The model under review builds one solid part; all positions refer to its coordinate system, in mm. Face numbers are marked on the shaded views. A direction names the side the tool comes from. Give positions to 0.01 mm unless a question says otherwise; leave off trailing zeros. Order: outer loops, then holes, each group sorted by start corner. A loop starts at its lowest first (then second) coordinate and runs counter-clockwise, first axis right, second up.
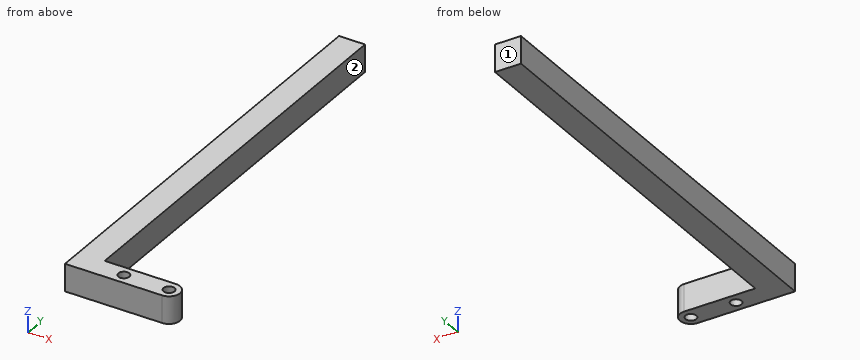
```python
from build123d import *

# Parameters (mm, degrees)
SKETCH_1_R      = 1
EXTRUDE_1_DEPTH = 5


with BuildPart() as part:
    # 草图1 → 凸台-拉伸1 (new body)
    with BuildSketch(Plane.XY):
        with BuildLine():
            Line((0, 2), (8.25, 2))
            ThreePointArc((8.25, 2), (10.25, 0), (8.25, -2))
            Line((8.25, -2), (-0.5, -2))
            Line((-0.5, -2), (-9.5, -2))
            Line((-9.5, -2), (-9.5, 78))
            Line((-9.5, 78), (-4.75, 78))
            Line((-4.75, 78), (-4.75, 2))
            Line((-4.75, 2), (0, 2))
        make_face()
        Circle(SKETCH_1_R, mode=Mode.SUBTRACT)
        with Locations((8.25, 0)):
            Circle(SKETCH_1_R, mode=Mode.SUBTRACT)
    extrude(amount=EXTRUDE_1_DEPTH)


solid = part.part
```
1. Take a section at C-C (z = 1.4). Write out the cut boundary in (x, y).
2. Take a section at D-D (x = 4.5). Write out the cut boundary in (y, z), and give its area (3 significant figures).
3. Insertion check: pin 1 (3 mm diameter, centred on y = 42, z = 2.5, fed in from +X); pin 2 (2.5 mm diameter, centred on x = 1, z = 2.5, fed in from +Y). Each pin has a flat end and moves straight along its axis. Give the tip position at first contact, or say it passes through.
4. Take a section at B-B (y = 0). Write out the cut boundary in (x, z).
5. For the marked faces 1 and 2, list the 3-axis set-ups (+Z, -Z, +X, -X, +Y, -Y) from which the entire face can be reached by the end or side of a thin tool; tool diameter is ignored.
6. Take a section at A-A (x = 0). Write out the cut boundary in (y, z), and give its area (3 significant figures).
7. To check wall thickness, follow line 1 (Y direction, x = 8.25, z = 1.95); line 2 (X direction, y = 19, z = 4.8); line 3 (Y direction, x = 4.25, z = 0.5). State the ranges of each line that lie inside material, in increasing order.
Answer:
1. outline: (-9.5, -2) - (8.25, -2) arc R2 ccw to (8.25, 2) - (-4.75, 2) - (-4.75, 78) - (-9.5, 78) - close; hole circle Ø2 at (0, 0); hole circle Ø2 at (8.25, 0)
2. outline: (-2, 0) - (2, 0) - (2, 5) - (-2, 5) - close
2. area: 20.0 mm2
3. pin 1: stops at x = -4.75
3. pin 2: stops at y = 2
4. outline: (-9.5, 0) - (-1, 0) - (-1, 5) - (-9.5, 5) - close; (1, 0) - (7.25, 0) - (7.25, 5) - (1, 5) - close; (9.25, 0) - (10.25, 0) - (10.25, 5) - (9.25, 5) - close
5. face 1: +Z, -Z, +X, -X, +Y
5. face 2: +Z, -Z, +X, +Y
6. outline: (-2, 0) - (-1, 0) - (-1, 5) - (-2, 5) - close; (1, 0) - (2, 0) - (2, 5) - (1, 5) - close
6. area: 10.0 mm2
7. line 1: y = -2 to -1, 1 to 2
7. line 2: x = -9.5 to -4.75
7. line 3: y = -2 to 2
